The model under review builds one solid part; all positions refer to its coordinate system, in mm. Coordinates: 2 decimals unless noted, no trailing zeros. Loops run counter-clockwise (first coordinate to the right, second up) from the corner with the lowest first, then second, coordinate; pieces in that order, holes last. Notation, with made-up numbers: M 79.25,66.25 L 90.25,66.25 A16 cw 90.25,75.25 Z; hole C -13,29.25 d6. An arc over 180 degrees is marked long. One line per item, written item: value.
```python
from build123d import *

# Parameters (mm, degrees)
SKETCH1_W               = 300
SKETCH1_H               = 220
BOSS_EXTRUDE1_DEPTH     = 5
SKETCH2_W               = 15
SKETCH2_H               = 88
CUT_EXTRUDE1_DEPTH      = 10
ESQUISSE2_R             = 2
ENL_V_MAT_EXTRU_1_DEPTH = 10
ESQUISSE4_W             = 16.5
ESQUISSE4_H             = 65
ENL_V_MAT_EXTRU_4_DEPTH = 5
ESQUISSE5_R             = 2
ENL_V_MAT_EXTRU_5_DEPTH = 10
ESQUISSE6_R             = 2.25
ENL_V_MAT_EXTRU_6_DEPTH = 10
ESQUISSE7_R             = 9
ENL_V_MAT_EXTRU_9_DEPTH = 10


with BuildPart() as part:
    # Sketch1 → Boss-Extrude1 (new body)
    with BuildSketch(Plane(origin=(0, 0, 0), x_dir=(1, 0, 0), z_dir=(0, 1, 0))):
        Rectangle(SKETCH1_W, SKETCH1_H)
    extrude(amount=BOSS_EXTRUDE1_DEPTH)

    # Sketch2 → Cut-Extrude1 (cut)
    with BuildSketch(Plane(origin=(0, 5, 0), x_dir=(1, 0, 0), z_dir=(0, 1, 0))):
        with Locations((-142.5, 0)):
            Rectangle(SKETCH2_W, SKETCH2_H)
        with Locations((142.5, 0)):
            Rectangle(SKETCH2_W, SKETCH2_H)
    extrude(amount=-CUT_EXTRUDE1_DEPTH, mode=Mode.SUBTRACT)

    # Esquisse2 → Enlèv. mat.-Extru.1 (cut)
    with BuildSketch(Plane(origin=(0, 5, 0), x_dir=(1, 0, 0), z_dir=(0, 1, 0))):
        with Locations(Location((-105.8, 27.4, 0), (0, 0, 270))):
            Circle(ESQUISSE2_R)
        with Locations(Location((-25.2, 27.4, 0), (0, 0, 270))):
            Circle(ESQUISSE2_R)
        with Locations(Location((-25.2, -27.4, 0), (0, 0, 90))):
            Circle(ESQUISSE2_R)
        with Locations(Location((-105.8, -27.4, 0), (0, 0, 90))):
            Circle(ESQUISSE2_R)
        with Locations(Location((25.2, -27.4, 0), (0, 0, 270))):
            Circle(ESQUISSE2_R)
        with Locations(Location((105.8, -27.4, 0), (0, 0, 270))):
            Circle(ESQUISSE2_R)
        with Locations(Location((25.2, 27.4, 0), (0, 0, 90))):
            Circle(ESQUISSE2_R)
        with Locations(Location((105.8, 27.4, 0), (0, 0, 90))):
            Circle(ESQUISSE2_R)
    extrude(amount=-ENL_V_MAT_EXTRU_1_DEPTH, mode=Mode.SUBTRACT)

    # Esquisse4 → Enlèv. mat.-Extru.4 (cut)
    with BuildSketch(Plane(origin=(0, 5, 0), x_dir=(1, 0, 0), z_dir=(0, 1, 0))):
        with Locations((0, 77.5)):
            Rectangle(ESQUISSE4_W, ESQUISSE4_H)
    extrude(amount=-ENL_V_MAT_EXTRU_4_DEPTH, mode=Mode.SUBTRACT)

    # Esquisse5 → Enlèv. mat.-Extru.5 (cut)
    with BuildSketch(Plane(origin=(0, 5, 0), x_dir=(1, 0, 0), z_dir=(0, 1, 0))):
        with Locations(Location((-14.16612842, 86.53761558, 0), (0, 0, 270))):
            Circle(ESQUISSE5_R)
        with Locations(Location((-14.16612842, 64.64560566, 0), (0, 0, 270))):
            Circle(ESQUISSE5_R)
    extrude(amount=-ENL_V_MAT_EXTRU_5_DEPTH, mode=Mode.SUBTRACT)

    # Esquisse6 → Enlèv. mat.-Extru.6 (cut)
    with BuildSketch(Plane(origin=(0, 5, 0), x_dir=(1, 0, 0), z_dir=(0, 1, 0))):
        with Locations(Location((-137, -80, 0), (0, 0, 270))):
            Circle(ESQUISSE6_R)
        with Locations(Location((-106, -80, 0), (0, 0, 270))):
            Circle(ESQUISSE6_R)
        with Locations(Location((106, -80, 0), (0, 0, 90))):
            Circle(ESQUISSE6_R)
        with Locations(Location((137, -80, 0), (0, 0, 90))):
            Circle(ESQUISSE6_R)
        with Locations(Location((137, 80, 0), (0, 0, 270))):
            Circle(ESQUISSE6_R)
        with Locations(Location((106, 80, 0), (0, 0, 270))):
            Circle(ESQUISSE6_R)
        with Locations(Location((-106, 80, 0), (0, 0, 90))):
            Circle(ESQUISSE6_R)
        with Locations(Location((-137, 80, 0), (0, 0, 90))):
            Circle(ESQUISSE6_R)
    extrude(amount=-ENL_V_MAT_EXTRU_6_DEPTH, mode=Mode.SUBTRACT)

    # Esquisse7 → Enlèv. mat.-Extru.9 (cut)
    with BuildSketch(Plane(origin=(0, 5, 0), x_dir=(1, 0, 0), z_dir=(0, 1, 0))):
        with Locations(Location((-121.5, 80, 0), (0, 0, 270))):
            Circle(ESQUISSE7_R)
        with Locations(Location((-121.5, -80, 0), (0, 0, 90))):
            Circle(ESQUISSE7_R)
        with Locations(Location((121.5, -80, 0), (0, 0, 270))):
            Circle(ESQUISSE7_R)
        with Locations(Location((121.5, 80, 0), (0, 0, 90))):
            Circle(ESQUISSE7_R)
    extrude(amount=-ENL_V_MAT_EXTRU_9_DEPTH, mode=Mode.SUBTRACT)


solid = part.part
```
(1) To check wall thickness, follow L1, parallel to X at y = 3.4, z = 27.4; L2, parallel to Z at x = 125.5, y = 3.2; L3, parallel to X at y = 2.45, z = -63. State the ranges of each line that lie inside material, in increasing order. Write a range as [from, to].
Checks:
L1: [-135, -107.8], [-103.8, -27.2], [-23.2, 23.2], [27.2, 103.8], [107.8, 135]
L2: [-110, -88.06], [-71.94, 71.94], [88.06, 110]
L3: [-150, -15.3], [-13.03, -8.25], [8.25, 150]
(2) Draft analysis for pull direction X (two halves, no side actions). For faces 1 (the face through (-124.203, 2.535, 71.416)), 2 (the face through (-2, 0, -2)), state which applies: pulls with the +X half, pulls with the -X half, needs draft (parallel to the pull), parting line crosses it, or undercut.
Checks:
face 1: undercut
face 2: needs draft
(3) Add section B-B on x = 121.5. State the section outline as (y, z) points, then the cut area to 3 significant figures.
Checks:
outline: M 0,-110 L 5,-110 L 5,-89 L 0,-89 Z; M 0,-71 L 5,-71 L 5,71 L 0,71 Z; M 0,89 L 5,89 L 5,110 L 0,110 Z
area: 920 mm^2
(4) Insertion check: pin 1 Ø20.5 at (x, z) = (-121.5, -80) entering from -Y; pin 2 Ø2.5 at (y, z) = (1.5, -1.5) entering from -X. Each pin has a flat end and moves straight along its axis. Give the tip position at first contact, or say it passes through.
Checks:
pin 1: y = 0
pin 2: x = -135
(5) Add section C-C on z = -39. State the section outline as (x, y) points.
Checks:
outline: M -135,0 L 135,0 L 135,5 L -135,5 Z
(6) Add section D-D on y = 1. State how many separate pieces and enclosed holes the cut face has, then the cut area to 3 significant figures.
Checks:
separate pieces: 1
enclosed holes: 22
area: 61,000 mm^2
(7) Add section A-A on z = -95.5. State the section outline as (x, y) points, then the cut area to 3 significant figures.
Checks:
outline: M -150,0 L -8.25,0 L -8.25,5 L -150,5 Z; M 8.25,0 L 150,0 L 150,5 L 8.25,5 Z
area: 1,420 mm^2
